Geometry: see drawing. Coordinates: mm, zero at the bounding-box minimum. Give positions to 0.01 mm unless a question says otherwise; leave off trailing zeros. Order: outer loops, then holes, each group sorted by start corner. A loop starts at its lowest first (then second) coordinate and runs counter-clockwise, first axis right, second up. Notation, with made-up numbers: (41.5, 30.25) - (64.5, 30.25) arc R25 ccw to (64.5, 58.25) - close; hole circle Ø9 at (-11, 31.5). An arc over 180 degrees is marked (long way). One line per item, written item: value.
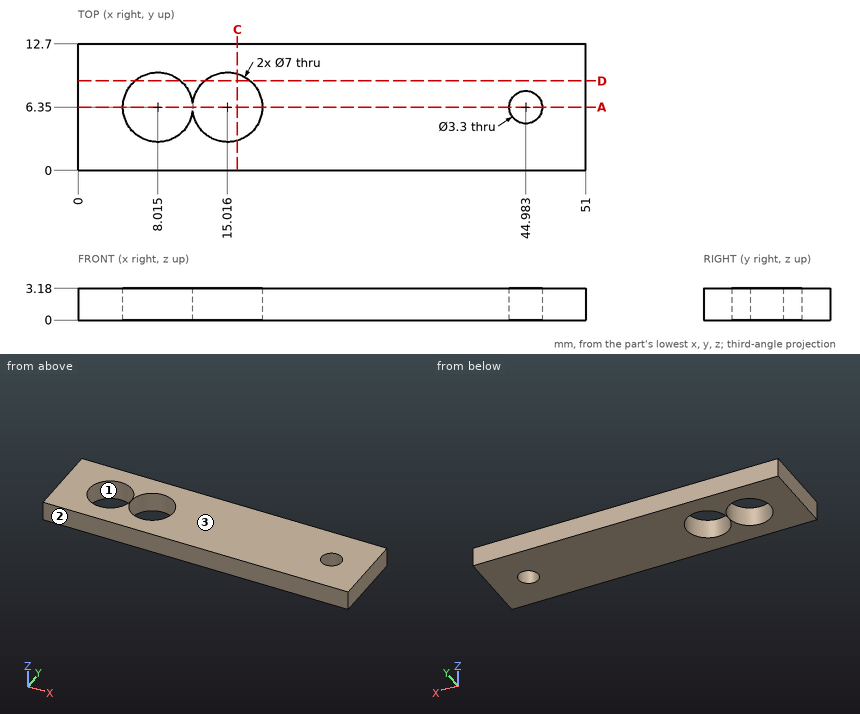
1) First-contact query: pin 1 (1 mm diameter, centred on x = 44.5, y = 4.5, fed in from -Z). Flat tip, straight axial feed; report the tip coordinate or a pass-through.
Answers below:
pin 1: z = 0
2) Section A-A, the plane y = 6.35. Count the separate pieces of the cut face and the enclosed holes in it, then the cut area to 3 significant figures.
Answers below:
separate pieces: 4
enclosed holes: 0
area: 107 mm^2
3) Section C-C, the plane x = 16. Return loops of the section in (y, z), then the cut area to 3 significant figures.
Answers below:
outline: (0, 0) - (2.99, 0) - (2.99, 3.18) - (0, 3.18) - close; (9.71, 0) - (12.7, 0) - (12.7, 3.18) - (9.71, 3.18) - close
area: 19.0 mm^2
4) Material intervals for line 1 along X through (y, z) = (8.25, 0.3) (1 decimal); line 2 along X through (y, z) = (4.5, 2.3) (1 decimal); line 3 along X through (y, z) = (7.5, 2.25) (1 decimal), sorted ascending.
Answers below:
line 1: 0 to 5.1, 11 to 12.1, 18 to 51
line 2: 0 to 5, 11 to 12, 18 to 51
line 3: 0 to 4.7, 11.3 to 11.7, 18.3 to 43.8, 46.2 to 51
5) Section D-D, the plane y = 9. Return loops of the section in (x, z), then the cut area to 3 significant figures.
Answers below:
outline: (0, 0) - (5.73, 0) - (5.73, 3.18) - (0, 3.18) - close; (10.3, 0) - (12.73, 0) - (12.73, 3.18) - (10.3, 3.18) - close; (17.3, 0) - (51, 0) - (51, 3.18) - (17.3, 3.18) - close
area: 133 mm^2
6) Mould query, pull axis Y, two halves, no side actions, for the marked faces 1, 2 and 3. Classes: released by +Y, released by -Y, zero draft, split by the parting line, or undercut.
Answers below:
face 1: undercut
face 2: released by -Y
face 3: zero draft
